Geometry check sheet. Reference: the model listing, model coordinates, mm. Give positions to 0.01 mm unless a question says otherwise; leave off trailing zeros. Loops run counter-clockwise (first coordinate to the right, second up) from the corner with the lowest first, then second, coordinate; pieces in that order, holes last.
1. Release check for a two-part mould opening along Y. For faces 1 (the flat face through (-3, -42, -166.05)), 2 (the cylindrical face through (190.764, 60.075, -156.658)), 3 (the flat face through (3.3, -3, -158.05)) record: +Y half, -Y half, draft (parallel to the pull), parting line (faces both ways), or undercut.
2. Cross-section at A-A, the plane z = -162.75. Record the cut outline in (x, y), plus the area to 3 significant figures.
3. Go/stop test with flat-tipped pins: pin 1 Ø5 at (x, y) = (0, 0) entering from -Z; pin 2 Ø2 at (y, z) = (31, -161.5) entering from +X; pin 3 Ø10 at (x, z) = (-33.5, -161.5) entering from -Y; pin 4 Ø8 at (x, z) = (-131.5, -158) entering from +Y. Record where each tip stops, or that it passes through.
4. Material ranges on L1, parallel to Y at x = 0, z = -155.5; L2, parallel to X at y = 179.5, z = -162.5; L3, parallel to Y at x = 73.5, z = -152.75, recorded low to high.
5. Cross-section at C-C, the plane x = 64. Record the cut outline in (y, z).
6. Cross-section at B-B, the plane y = -169.5. Record the cut outline in (x, z), plus the area to 3 significant figures.
from build123d import *

# Parameters (mm, degrees)
CYLINDER006_R     = 200
CYLINDER006_DEPTH = 19.05
POCKET045_DEPTH   = 8
SKETCH106_R       = 4.2
HOLE037_DEPTH     = 11.051


with BuildPart() as part:
    # Cylinder006 → Cylinder006 (join)
    with BuildSketch(Plane.XY.offset(-19.05)):
        Circle(CYLINDER006_R)
    extrude(amount=CYLINDER006_DEPTH)

    # Sketch105 (on Face3 of Cylinder006) → Pocket045 (cut)
    with BuildSketch(Plane(origin=(0, 0, -19.05), x_dir=(1, 0, 0), z_dir=(0, 0, -1))):
        Polygon((3.810512, -6.6), (7.621024, 0), (3.810512, 6.6), (-3.810512, 6.6), (-7.621024, 0), (-3.810512, -6.6), align=None)
    extrude(amount=-POCKET045_DEPTH, mode=Mode.SUBTRACT)

    # Sketch106 (on Face10 of Pocket045) → Hole037 (cut, through all)
    with BuildSketch(Plane(origin=(0, 0, -11.05), x_dir=(1, 0, 0), z_dir=(0, 0, -1))):
        Circle(SKETCH106_R)
    extrude(amount=-HOLE037_DEPTH, mode=Mode.SUBTRACT)


with BuildPart() as part_1:
    # Body022020 placement: moved
    add(part.part.moved(Location((0, 0, -147))))


solid = part_1.part
Result:
1. face 1: draft
1. face 2: parting line
1. face 3: undercut
2. outline: circle Ø400 at (0, 0); hole (-7.62, 0) - (-3.81, -6.6) - (3.81, -6.6) - (7.62, 0) - (3.81, 6.6) - (-3.81, 6.6) - close
2. area: 126,000 mm2
3. pin 1: passes through
3. pin 2: stops at x = 197.74
3. pin 3: stops at y = -197.96
3. pin 4: stops at y = 154.09
4. L1: y = -200 to -4.2, 4.2 to 200
4. L2: x = -88.2 to 88.2
4. L3: y = -186 to 186
5. outline: (-189.48, -166.05) - (189.48, -166.05) - (189.48, -147) - (-189.48, -147) - close
6. outline: (-106.16, -166.05) - (106.16, -166.05) - (106.16, -147) - (-106.16, -147) - close
6. area: 4,040 mm2
